Geometry: final body of the model. Coordinates: model frame, mm. A direction names the side the tool comes from. Give positions to 0.01 mm unless a question says otherwise; leave off trailing zeros. Order: outer loops, then holes, each group sorted by start corner. A loop starts at its lowest first (then second) coordinate and runs counter-clockwise, first axis right, second up. Notation, with made-up numbers: (21, -35.5) - (37, -35.5) arc R16 cw to (37, -8.5) - close; hole circle Ø8 at (43, 69.25). An arc over 180 degrees is marked (long way). One line per item, written item: value.
```python
from build123d import *

# Parameters (mm, degrees)
CROQUIS1_W              = 200
CROQUIS1_H              = 200
SALIENTE_EXTRUIR1_DEPTH = 10
CORTAR_EXTRUIR2_DEPTH   = 10
CORTAR_EXTRUIR3_DEPTH   = 8
CROQUIS6_R              = 1.5
CORTAR_EXTRUIR4_DEPTH   = 32
VACIADO1_DEPTH          = 8


# Read off the part's stored shape, not the designer's step: Vaciado1
with BuildPart() as part:
    # Croquis1 → Saliente-Extruir1 (new body)
    with BuildSketch(Plane(origin=(0, 0, 0), x_dir=(1, 0, 0), z_dir=(0, 1, 0))):
        Rectangle(CROQUIS1_W, CROQUIS1_H)
    extrude(amount=SALIENTE_EXTRUIR1_DEPTH)

    # Croquis3 → Cortar-Extruir2 (cut)
    with BuildSketch(Plane(origin=(0, 10, 0), x_dir=(1, 0, 0), z_dir=(0, 1, 0))):
        with BuildLine():
            add(Edge.make_bspline(
                [(-54.658905902, 100), (-5.437672215, 0.742753657), (-54.658905902, -100)],
                knots=[0, 0, 0, 1, 1, 1], degree=2))
            Line((-54.658905902, 100), (-100, 100))
            Line((-100, 100), (-100, -100))
            Line((-100, -100), (-54.658905902, -100))
        make_face()
        with BuildLine():
            Line((100, 100), (18.719386755, 100))
            add(Edge.make_bspline(
                [(18.719386755, 100), (67.218637457, 0), (18.719386755, -100)],
                knots=[0, 0, 0, 1, 1, 1], degree=2))
            Line((18.719386755, -100), (100, -100))
            Line((100, -100), (100, 100))
        make_face()
    extrude(amount=-CORTAR_EXTRUIR2_DEPTH, mode=Mode.SUBTRACT)

    # Croquis4 → Cortar-Extruir3 (cut)
    with BuildSketch(Plane(origin=(0, 10, 0), x_dir=(1, 0, 0), z_dir=(0, 1, 0))):
        Polygon((-50.296578731, -90.149033959), (-40.296578731, -90.149033959), (-40.296578731, -100.149033959), (-50.296578731, -100.149033959), (-58.120283929, -100.149033959), align=None)
        Polygon((8.836094338, -90.149033959), (18.836094338, -90.149033959), (23.704036403, -90.149033959), (18.836094338, -100.149033959), (8.836094338, -100.149033959), align=None)
        Polygon((8.836094338, 90.149033959), (8.836094338, 100.149033959), (18.836094338, 100.149033959), (23.704036403, 90.149033959), (18.836094338, 90.149033959), align=None)
        Polygon((-58.120283929, 100.149033959), (-50.296578731, 90.149033959), (-40.296578731, 90.149033959), (-40.296578731, 100.149033959), (-50.296578731, 100.149033959), align=None)
    extrude(amount=-CORTAR_EXTRUIR3_DEPTH, mode=Mode.SUBTRACT)

    # Croquis6 → Cortar-Extruir4 (cut)
    with BuildSketch(Plane(origin=(0, 2, 0), x_dir=(1, 0, 0), z_dir=(0, 1, 0))):
        with Locations(Location((-46.580021795, -95.07451698, 0), (0, 0, 270))):
            Circle(CROQUIS6_R)
        with Locations(Location((14.358607989, -95.07451698, 0), (0, 0, 270))):
            Circle(CROQUIS6_R)
        with Locations(Location((14.358607989, 95.07451698, 0), (0, 0, 270))):
            Circle(CROQUIS6_R)
        with Locations(Location((-46.580021795, 95.07451698, 0), (0, 0, 270))):
            Circle(CROQUIS6_R)
    extrude(amount=-CORTAR_EXTRUIR4_DEPTH, mode=Mode.SUBTRACT)

    # Vaciado1 outline → Vaciado1 (cut)
    with BuildSketch(Plane(origin=(0, 0, 0), x_dir=(1, 0, 0), z_dir=(0, 1, 0))):
        with BuildLine():
            Line((-38.296578731, 88.149033959), (-46.954714444, 88.14903419))
            add(Edge.make_bspline(
                [(-46.954714444, 88.14903419), (-39.391707249, 70.655852329), (-33.505222898, 53.123612665), (-29.298629275, 35.553220346), (-26.77560099, 17.947129894), (-25.939405083, 0.309621467), (-26.791931975, -17.352344743), (-29.330747185, -35.032202144), (-33.552462911, -52.726080621), (-39.453418895, -70.431901676), (-47.030358691, -88.149034179)],
                knots=[0.063666004, 0.063666004, 0.063666004, 0.063666004, 0.063666004, 0.063666004, 0.063666004, 0.063666004, 0.063666004, 0.063666004, 0.063666004, 0.937249877, 0.937249877, 0.937249877, 0.937249877, 0.937249877, 0.937249877, 0.937249877, 0.937249877, 0.937249877, 0.937249877, 0.937249877], degree=10))
            Line((-47.030358691, -88.149034179), (-38.296578731, -88.149033959))
            Line((-38.296578731, -88.149033959), (-38.296578731, -98))
            Line((-38.296578731, -98), (6.836094338, -98))
            Line((6.836094338, -98), (6.836094338, -88.149033959))
            Line((6.836094338, -88.149033959), (21.949825856, -88.149033757))
            add(Edge.make_bspline(
                [(21.949825856, 88.149033757), (30.411471368, 68.532743192), (36.750179646, 48.933917862), (40.970725224, 29.351479613), (43.07830794, 9.781812592), (43.07830794, -9.781812592), (40.970725224, -29.351479613), (36.750179646, -48.933917862), (30.411471368, -68.532743192), (21.949825856, -88.149033757)],
                knots=[0.055294031, 0.055294031, 0.055294031, 0.055294031, 0.055294031, 0.055294031, 0.055294031, 0.055294031, 0.055294031, 0.055294031, 0.944705969, 0.944705969, 0.944705969, 0.944705969, 0.944705969, 0.944705969, 0.944705969, 0.944705969, 0.944705969, 0.944705969], degree=9))
            Line((21.949825856, 88.149033757), (6.836094338, 88.149033959))
            Line((6.836094338, 88.149033959), (6.836094338, 98))
            Line((6.836094338, 98), (-38.296578731, 98))
            Line((-38.296578731, 98), (-38.296578731, 88.149033959))
        make_face()
    extrude(amount=VACIADO1_DEPTH, mode=Mode.SUBTRACT)


solid = part.part
```
1) First-contact query: pin 1 (5 mm diameter, centred on x = 17, z = 96.5, fed in from +Y); pin 2 (4 mm diameter, centred on y = 3, z = 26, fed in from +X); pin 3 (2 mm diameter, centred on x = 17, y = 8.5, fed in from -Z). Flat tips, straight axial feed; report the tip coordinate or a pass-through.
Answers below:
pin 1: y = 2
pin 2: x = 41.57
pin 3: z = -90.15
2) Material intervals for line 1 along Z through (x, y) = (-5, 0.75); line 2 along Z through (x, y) = (12, 1.75); line 3 along X through (y, z) = (7, 36), sorted ascending.
Answers below:
line 1: -100 to -98, 98 to 100
line 2: -100 to -88.15, 88.15 to 100
line 3: -33.3 to -31.26, 37.8 to 39.83
3) Set-up query: faces 1 (the face through (16, 6, 90.149)), 2 (the face through (-43, 4, -88.149)), 3 (the face through (-45, 6, 90.149)), 4 (the face through (8.836, 6, -95)), 5 (the face through (-48, 2, -96)). Return all of +Z, -Z, +X, -X, +Y, -Y with unobstructed straight access to the full face (end or side cutting, diameter ignored); none if empty.
Answers below:
face 1: +Z, +X, +Y
face 2: -Y
face 3: +Z, -X, +Y
face 4: -Z, +X, +Y
face 5: -Z, -X, +Y
4) Section A-A, the plane x = -20.5. Return loops of the section in (y, z).
Answers below:
outline: (0, -100) - (10, -100) - (10, 100) - (0, 100) - (0, 98) - (8, 98) - (8, -98) - (0, -98) - close
